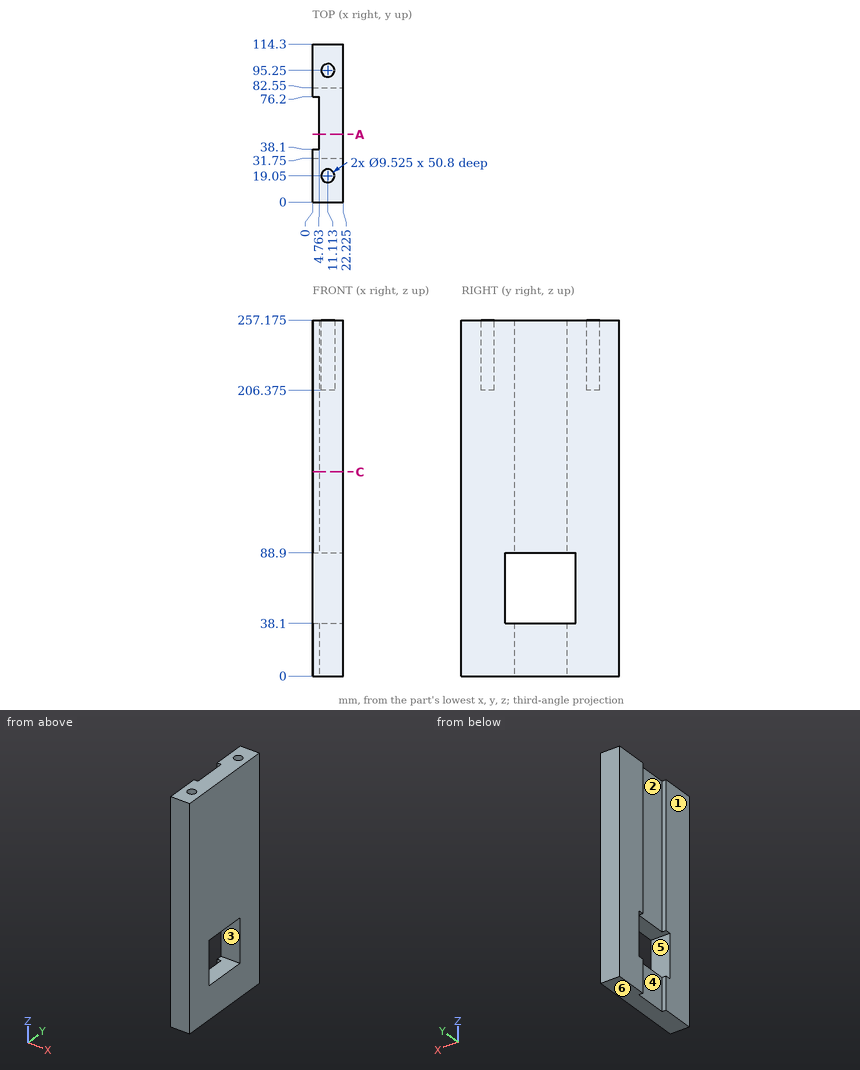
Answer from the drawing. Dimensions are ordinates in mm from the lowest x, y and z of the part. A direction names the side the tool comes from. Give positions to 0.01 mm unless a question says otherwise; leave off trailing zeros. Loops run counter-clockwise (first coordinate to the right, second up) from the corner with the lowest first, then second, coordinate; pieces in that order, holes last.
Item 1: For the marked faces 1, 2 and 3, determine the directions among +Z, -Z, +X, -X, +Y, -Y from which every point of the face is accessible in a straight line to the end or side of a thin tool.
Item 2: The part is cut by section A-A (y = 49). Write down the section's boundary in (x, z) (1 decimal).
Item 3: Find the intervals of material crossed by line 1 along Y through (x, z) = (5.25, 80.5); line 2 along X through (y, z) = (95, 221) (1 decimal); line 3 along Y through (x, z) = (3, 16), in increasing order.
Item 4: Each of these flat-tipped pins is pushed along its axis until it touches: pin 1 Ø5.5 at (x, y) = (11.11, 19.05) entering from +Z (1 decimal); pin 2 Ø19 at (y, z) = (64, 179.5) entering from -X. Where does it stop, or does it pass through?
Item 5: The part is cut by section C-C (z = 147.5). Write down the section's boundary in (x, y) (1 decimal), and give its area (3 significant figures).
Item 6: The mould has two halves that part along Z. Classify the marked faces 4, 5 and 6: released by +Z, released by -Z, zero draft, split by the parting line, or undercut.
Taken from the geometry:
1. face 1: +Z, -Z, -X, +Y, -Y
1. face 2: +Z, -Z, -X
1. face 3: +X, -X
2. outline: (4.8, 0) - (22.2, 0) - (22.2, 38.1) - (4.8, 38.1) - close; (4.8, 88.9) - (22.2, 88.9) - (22.2, 257.2) - (4.8, 257.2) - close
3. line 1: y = 0 to 31.75, 82.55 to 114.3
3. line 2: x = 0 to 6.4, 15.9 to 22.2
3. line 3: y = 0 to 38.1, 76.2 to 114.3
4. pin 1: stops at z = 206.4
4. pin 2: stops at x = 4.76
5. outline: (0, 0) - (22.2, 0) - (22.2, 114.3) - (0, 114.3) - (0, 76.2) - (4.8, 76.2) - (4.8, 38.1) - (0, 38.1) - close
5. area: 2,360 mm2
6. face 4: zero draft
6. face 5: undercut
6. face 6: released by -Z
